Autodesk Inventor part; units mm, degrees
ref_plane "YZ Plane" through (0, 0, 0) normal (1, 0, 0) x (0, 1, 0)
ref_plane "XZ Plane" through (0, 0, 0) normal (0, 1, 0) x (-1, 0, 0)
ref_plane "XY Plane" through (0, 0, 0) normal (0, 0, 1) x (1, 0, 0)
sketch "Sketch1" plane through (0, 0, 0) normal (0, 0, 1) x (1, 0, 0)
  line L0 (0, 0) -> (0, 20)
  line L1 (0, 0) -> (20, 0)
  arc A0 (20, 0) -> (0, 20) centre (0, 0) ccw
  line L2 (0, -4.8284) -> (0, 28.9706)
  dimension "d2" = 20
revolve "Revolution1" add sketch "Sketch1" angle 360 about axis through (0, -10, 0) along (0, 1, 0)
sketch "Sketch4" plane through (0, 0, 0) normal (0, -1, 0) x (1, 0, 0)
  point P0 (0, 0)
  point P1 (0, 0)
hole "Hole2" at (0, 0, 0) direction (0, 1, 0) diameter 3.242 depth 11.8 tip angle 118
shell "Shell2" thickness 5 removed faces 1 at (13.676, 0, 1.6606)
properties part number "Ball_Upper Half" material "Nylon 6/6"
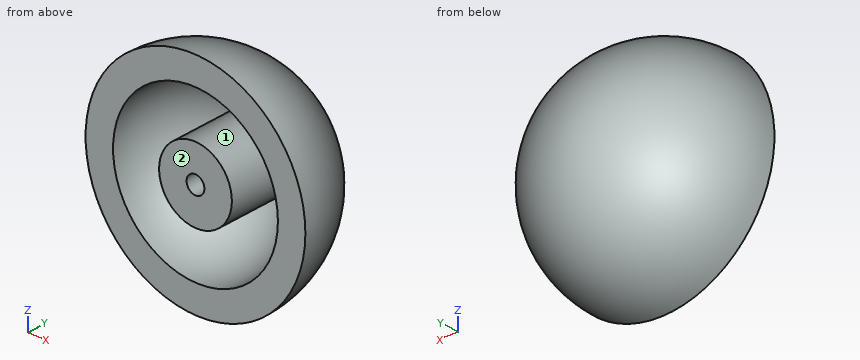
Verification items for the finished model (mm, model axes). Face numbers are marked on the shaded views. Round coordinates to 2 decimals unless told otherwise and drop trailing zeros. Write each loop counter-clockwise with the first axis right and the second up, starting at its lowest first coordinate (ties: lowest second). Pieces come first, ordered by that corner, then holes. Notation, with made-up numbers: (61, 62.25) - (71, 62.25) arc R11 ccw to (71, 75.25) - close; hole circle Ø1 at (66.25, -34.5). An arc over 180 degrees is marked (long way). Answer as a JSON object with one key per item and string values. Group by question number.
Q1. Section check C-C, the plane y = 18. Enter the section's corners in (x, z).
Q2. Section check B-B, the plane z = -3. Enter the section's corners in (x, y).
Q3. Section check D-D, the plane z = -11. Enter the section's corners in (x, y), plus the area to 3 significant figures.
Q4. Go/stop test with flat-tipped pins: pin 1 Ø3 at (x, y) = (-7.5, 4) entering from -Z (3 decimals); pin 2 Ø1 at (x, y) = (-4.5, 4.5) entering from -Z; pin 3 Ø12 at (x, y) = (10.5, 4.5) entering from +Z. Record where each tip stops, or that it passes through.
Q5. Mould release check, pull along Z, two halves, no side actions. Record for the marked faces 1 and 2: released by +Z, released by -Z, zero draft, split by the parting line, or undercut.
Q6. Section check A-A, the plane x = 5.5. Enter the section's corners in (y, z), plus the area to 3 significant figures.
Q7. Thickness scan on line 1 (X direction, y = 8.25, z = 0); line 2 (X direction, y = 2.5, z = 0); line 3 (Z direction, x = 0, y = 9). Record the ranges inside material, lowest first.
Found:
{
 "1": {"outline": "circle Ø17.44 at (0, 0)"},
 "2": {"outline": "(-19.77, 0) - (-14.7, 0) arc R14.7 cw to (-5.9, 13.46) - (-5.9, 0) - (5.9, 0) - (5.9, 13.46) arc R14.7 cw to (14.7, 0) - (19.77, 0) arc R19.77 ccw to start"},
 "3": {"outline": "(-16.7, 0) - (-10.2, 0) arc R10.2 cw to (10.2, 0) - (16.7, 0) arc R16.7 ccw to start", "area": "275 mm^2"},
 "4": {"pin 1": "stops at z = -18.735", "pin 2": "stops at z = -19.12", "pin 3": "stops at z = 19.25"},
 "5": {"face 1": "undercut", "face 2": "zero draft"},
 "6": {"outline": "(0, -19.23) arc R19.23 ccw to (0, 19.23) - (0, 13.96) arc R13.96 cw to (13.46, 3.69) - (0, 3.69) - (0, -3.69) - (13.46, -3.69) arc R13.96 cw to (0, -13.96) - close", "area": "377 mm^2"},
 "7": {"line 1": "x = -18.22 to -12.53, -6.62 to -1.62, 1.62 to 6.62, 12.53 to 18.22", "line 2": "x = -19.84 to -14.79, -6.62 to -1.62, 1.62 to 6.62, 14.79 to 19.84", "line 3": "z = -17.86 to -12, -6.62 to -1.62, 1.62 to 6.62, 12 to 17.86"}
}
